Input: part model. Units: mm. Frame: model coordinates. A direction names the side the tool comes from. Give positions to 0.01 mm unless a question says otherwise; leave off trailing zeros. Write each loop counter-clockwise with the first axis right and the second up, starting at its lowest first coordinate (ties: lowest second). Pieces come first, ordered by that corner, then holes. Notation, with made-up numbers: (29.5, 8) - (71.5, 8) arc R34 ccw to (71.5, 40) - close; hole circle Ø4 at (59, -16). An arc over 180 degrees is marked (long way). Use a Markdown table: item, result. Add a question column.
1. Pin query (flat end, axial travel): pin 1 (6 mm diameter, centred on x = -20, y = 5.5, fed in from -Z). Return the tip coordinate at first contact, or that it passes through.
2. Material intervals for probe 1 along X at (y, z) = (-1.25, 0.3) (3 decimals), sorted ascending.
3. Mould query, pull axis X, two halves, no side actions, for faces 3 (the flat face through (0, -10.787, 2)), 4 (the flat face through (-25, -1, 2)), 5 (the flat face through (-14, -0.562, 2)), 6 (the flat face through (-15.025, -2, 2)). Classes: released by +X, released by -X, zero draft, split by the parting line, or undercut.
4. Set-up query: faces 1 (the flat face through (-12.975, -2, 2)), 2 (the flat face through (0, -1, 0)). Return all of +Z, -Z, +X, -X, +Y, -Y with unobstructed straight access to the full face (end or side cutting, diameter ignored); none if empty.
5. Section query A-A, the plane y = -1. Return loops of the section in (x, z) (3 decimals), plus the area to 3 significant figures.
```python
from build123d import *

# Parameters (mm, degrees)
SKETCH2_W           = 2.05
SKETCH2_H           = 2.05
BOSS_EXTRUDE1_DEPTH = 3.175


with BuildPart() as part:
    # Sketch2 → Boss-Extrude1 (new body)
    with BuildSketch(Plane.XY):
        Polygon((-25, -10.7874943), (25, -10.7874943), (25, -1), (25, 1), (25, 7.6124943), (22.5, 7.6124943), (20.5, 7.6124943), (18, 7.6124943), (-18, 7.6124943), (-20.5, 7.6124943), (-22.5, 7.6124943), (-25, 7.6124943), (-25, 1), (-25, -1), align=None)
        with Locations((-14, -1.5874943)):
            Rectangle(SKETCH2_W, SKETCH2_H, mode=Mode.SUBTRACT)
        with Locations((14, -1.5874943)):
            Rectangle(SKETCH2_W, SKETCH2_H, mode=Mode.SUBTRACT)
    extrude(amount=BOSS_EXTRUDE1_DEPTH)


solid = part.part
```
Result sheet:
| question | item | result |
|---|---|---|
| 1 | pin 1 | stops at z = 0 |
| 2 | probe 1 | x = -25 to -15.025, -12.975 to 12.975, 15.025 to 25 |
| 3 | face 3 | zero draft |
| 3 | face 4 | released by -X |
| 3 | face 5 | undercut |
| 3 | face 6 | undercut |
| 4 | face 1 | +Z, -Z |
| 4 | face 2 | -Z, +X, -X, +Y, -Y |
| 5 | outline | (-25, 0) - (-15.025, 0) - (-15.025, 3.175) - (-25, 3.175) - close; (-12.975, 0) - (12.975, 0) - (12.975, 3.175) - (-12.975, 3.175) - close; (15.025, 0) - (25, 0) - (25, 3.175) - (15.025, 3.175) - close |
| 5 | area | 146 mm² |
